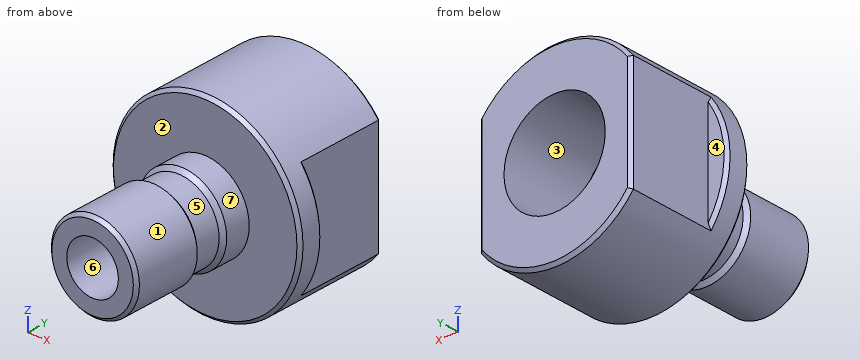
from build123d import *

# Parameters (mm, degrees)
SKETCH2_W          = 20.13485227
SKETCH2_H          = 29.427861008
SKETCH2_W_2        = 12
SKETCH2_H_2        = 20.553456266
CUT_EXTRUDE1_DEPTH = 6.89
CHAMFER2_SIZE      = 0.254
CHAMFER4_SIZE      = 0.254
CHAMFER5_SIZE      = 0.254


with BuildPart() as part:
    # Sketch1 → Revolve1 (revolve)
    with BuildSketch(Plane.XY):
        Polygon((7.5, 0), (7.5, -8.89), (3.475, -8.89), (3.475, -10.89), (3.159135291, -11.205864709), (3.159135291, -13.185864709), (3.475, -13.501729418), (3.475, -18.89), (2.0381, -18.89), (2.0381, -8.0269), (3.175, -6.89), (4, -6.89), (4, 0), align=None)
    revolve(axis=Axis((0, 0, 0), (0, -1, 0)))

    # Sketch2 → Cut-Extrude1 (cut)
    with BuildSketch(Plane(origin=(0, 0, 0), x_dir=(1, 0, 0), z_dir=(0, 1, 0))):
        Rectangle(SKETCH2_W, SKETCH2_H)
        Rectangle(SKETCH2_W_2, SKETCH2_H_2, mode=Mode.SUBTRACT)
    extrude(amount=-CUT_EXTRUDE1_DEPTH, mode=Mode.SUBTRACT)

    # Chamfer2
    chamfer2_edges = [part.edges().sort_by_distance(p)[0] for p in [
        (-3.475, -18.89, 0),
        (-7.5, -8.89, 0),
    ]]
    chamfer(chamfer2_edges, length=CHAMFER2_SIZE)

    # Chamfer4
    chamfer4_edges = [part.edges().sort_by_distance(p)[0] for p in [
        (0, 0, -7.5),
        (0, 0, 7.5),
        (6, 0, 0),
        (-6, 0, 0),
    ]]
    chamfer(chamfer4_edges, length=CHAMFER4_SIZE)

    # Chamfer5
    chamfer5_edges = [part.edges().sort_by_distance(p)[0] for p in [
        (-7.5, -6.89, 0),
        (7.115124735, -6.89, 2.371708245),
    ]]
    chamfer(chamfer5_edges, length=CHAMFER5_SIZE)


solid = part.part
Model file for the job. Use its own axes, mm. Face numbers are marked on the shaded views. A direction names the side the tool comes from. Give positions to 0.01 mm unless a question says otherwise; leave off trailing zeros. Loops run counter-clockwise (first coordinate to the right, second up) from the corner with the lowest first, then second, coordinate; pieces in that order, holes last.
1) Saw through at B-B (y = -6.5). Write the cut outline in (x, z), plus the area to 3 significant figures.
2) Wall check: line 1 (Z direction, x = 0, y = -4); line 2 (Z direction, x = 0, y = -12.25); line 3 (Y direction, x = -6.5, z = -1). Give the ranges that are in metal, low to high.
3) Saw through at D-D (y = -9.5). Write the cut outline in (x, z) (3 decimals).
4) Tool access for the marked faces 4, 5, 6 and 7: list every direction of +Z, -Z, +X, -X, +Y, -Y with a clear straight run to the whole face (end or side of a thin tool).
5) Pull direction X, two halves, no side cores. Call the marked faces 1, 2 and 3: +X half, -X half, draft (parallel to the pull), parting line (faces both ways), or undercut.
6) Flat gauge pins, fed straight in: pin 1 Ø8 at (y, z) = (-15, -1.5) entering from -X (3 decimals); pin 2 Ø2 at (y, z) = (-3.5, -0.5) entering from +X; pin 3 Ø3 at (x, y) = (-3.5, -4) entering from -Z; pin 4 Ø9 at (x, z) = (1.5, 0.5) entering from +Y. Where does each tip first touch, or does it go through?
7) Saw through at C-C (y = -12). Write the cut outline in (x, z), plus the area to 3 significant figures.
Answer block:
1. outline: (-6, -4.5) arc R7.5 ccw to (6, -4.5) - (6, 4.5) arc R7.5 ccw to (-6, 4.5) - close; hole circle Ø8 at (0, 0)
1. area: 108 mm2
2. line 1: z = -7.5 to -4, 4 to 7.5
2. line 2: z = -3.16 to -2.04, 2.04 to 3.16
2. line 3: y = -8.89 to -6.89
3. outline: circle Ø6.95 at (0, 0); hole circle Ø4.076 at (0, 0)
4. face 4: +Z, -Z, -X, +Y
4. face 5: none
4. face 6: +Y, -Y
4. face 7: -Y
5. face 1: parting line
5. face 2: draft
5. face 3: undercut
6. pin 1: stops at x = -3.475
6. pin 2: stops at x = 6
6. pin 3: stops at z = -7.23
6. pin 4: stops at y = 0
7. outline: circle Ø6.32 at (0, 0); hole circle Ø4.08 at (0, 0)
7. area: 18.3 mm2
